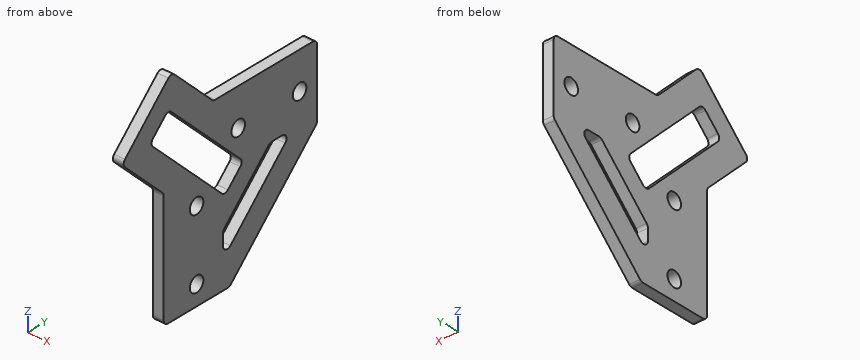
```python
from build123d import *

# Parameters (mm, degrees)
SKETCH_1_R      = 1.55
EXTRUDE_1_DEPTH = 2.2
FILLET_1_R      = 1


with BuildPart() as part:
    # 草图1 → 凸台-拉伸1 (new body)
    with BuildSketch(Plane(origin=(0, 0, 0), x_dir=(0, 0, -1), z_dir=(1, 0, 0))):
        Polygon((11.313708499, 0), (35, 0), (35, 15), (15, 35), (0, 35), (0, 11.313708499), (-9.545941546, 1.767766953), (1.767766953, -9.545941546), align=None)
        with Locations((7.5, 31)):
            Circle(SKETCH_1_R, mode=Mode.SUBTRACT)
        with Locations((7.5, 17)):
            Circle(SKETCH_1_R, mode=Mode.SUBTRACT)
        with Locations(Location((31, 7.5, 0), (0, 0, 180))):
            Circle(SKETCH_1_R, mode=Mode.SUBTRACT)
        with Locations(Location((17, 7.5, 0), (0, 0, 180))):
            Circle(SKETCH_1_R, mode=Mode.SUBTRACT)
        Polygon((13.939339828, 18.181980515), (18.181980515, 13.939339828), (1.060660172, -3.181980515), (-3.181980515, 1.060660172), align=None, mode=Mode.SUBTRACT)
        Polygon((13.5, 29.428932188), (13.5, 24.278174593), (24.278174593, 13.5), (29.428932188, 13.5), align=None, mode=Mode.SUBTRACT)
    extrude(amount=EXTRUDE_1_DEPTH)

    # 圆角1
    fillet_1_edges = [part.edges().sort_by_distance(p)[0] for p in [
        (1.1, 35, 0),
        (1.1, 35, -15),
        (1.1, 15, -35),
        (1.1, 0, -35),
        (1.1, 0, -11.313708499),
        (1.1, -9.545941546, -1.767766953),
        (1.1, 1.767766953, 9.545941546),
        (1.1, 11.313708499, 0),
        (1.1, 18.181980515, -13.939339828),
        (1.1, 1.060660172, 3.181980515),
        (1.1, -3.181980515, -1.060660172),
        (1.1, 13.939339828, -18.181980515),
        (1.1, 13.5, -24.278174593),
        (1.1, 13.5, -29.428932188),
        (1.1, 29.428932188, -13.5),
        (1.1, 24.278174593, -13.5),
    ]]
    fillet(fillet_1_edges, radius=FILLET_1_R)


solid = part.part
```
The model under review builds one solid part; all positions refer to its coordinate system, in mm. Coordinates: 2 decimals unless noted, no trailing zeros. Write each loop counter-clockwise with the first axis right and the second up, starting at its lowest first coordinate (ties: lowest second). Pieces come first, ordered by that corner, then holes. Notation, with made-up numbers: (67, -5.5) - (99, -5.5) arc R24 cw to (99, 19.5) - close; hole circle Ø7 at (34.25, 73). An arc over 180 degrees is marked (long way). Answer in a Markdown table with one row per item. Add a question column.
Q1. Consider section C-C on y = 7.5. Give the boundary of the cut face in (x, z).
Q2. To check wall thickness, follow line 1 along Y through (x, z) = (1.5, -7.5); line 2 along Y through (x, z) = (1.15, -17); line 3 along Z through (x, y) = (0.95, 17.5). State the ranges of each line that lie inside material, in increasing order. Write a range as from..to.
Q3. Consider section D-D on z = -8.5. Give the boundary of the cut face in (x, y), then the cut area to 3 significant figures.
Q4. Consider section B-B on z = -31. Give the boundary of the cut face in (x, y), then the cut area to 3 significant figures.
Q5. Clearance check with flat-ended pins moving along their axes: pin 1 (0.7 mm diameter, centred on x = 0.5, z = -26.5, fed in from +Y); pin 2 (1.1 mm diameter, centred on x = 1.5, y = 25, fed in from +Z). State where each tip first meets the part, or that it passes through.
Q6. Consider section A-A on y = 31. Give the boundary of the cut face in (x, z), then the cut area to 3 significant figures.
Answers below:
| question | item | result |
|---|---|---|
| 1 | outline | (0, -35) - (2.2, -35) - (2.2, -32.55) - (0, -32.55) - close; (0, -29.45) - (2.2, -29.45) - (2.2, -18.55) - (0, -18.55) - close; (0, -15.45) - (2.2, -15.45) - (2.2, -11.74) - (0, -11.74) - close; (0, -3.26) - (2.2, -3.26) - (2.2, 3.81) - (0, 3.81) - close |
| 2 | line 1 | -3.81..3.26, 11.74..15.45, 18.55..29.45, 32.55..35 |
| 2 | line 2 | 0..5.95, 9.05..12.76, 15.12..20.78, 25.93..33 |
| 2 | line 3 | -32.5..-25.43, -20.28..-14.62, -13.26..-8.97, -6.03..0 |
| 3 | outline | (0, -2.81) - (2.2, -2.81) - (2.2, 4.26) - (0, 4.26) - close; (0, 12.74) - (2.2, 12.74) - (2.2, 15.82) - (0, 15.82) - close; (0, 18.18) - (2.2, 18.18) - (2.2, 29.82) - (0, 29.82) - close; (0, 32.18) - (2.2, 32.18) - (2.2, 35) - (0, 35) - close |
| 3 | area | 54.1 mm² |
| 4 | outline | (0, 0) - (2.2, 0) - (2.2, 5.95) - (0, 5.95) - close; (0, 9.05) - (2.2, 9.05) - (2.2, 19) - (0, 19) - close |
| 4 | area | 35.0 mm² |
| 5 | pin 1 | y = 23.85 |
| 5 | pin 2 | z = 0 |
| 6 | outline | (0, -19) - (2.2, -19) - (2.2, -9.05) - (0, -9.05) - close; (0, -5.95) - (2.2, -5.95) - (2.2, 0) - (0, 0) - close |
| 6 | area | 35.0 mm² |
